The figure shows three views and two pictorial views of one solid part (mm, origin at its lowest corner). Answer the questions. Coordinates: 2 decimals unless noted, no trailing zeros. Loops run counter-clockwise (first coordinate to the right, second up) from the corner with the lowest first, then second, coordinate; pieces in that order, holes last. Notation, with made-up numbers: (76, -20) - (87, -20) arc R21 cw to (87, 16) - close; hole circle Ø9 at (32.5, 58). An arc over 180 degrees is marked (long way). Return JSON: item names as keys, results as strings. Group by question number.
1. Find the intervals of material crossed by line 1 along Z through (x, y) = (76.2, 5); line 2 along X through (y, z) = (4.75, 25.4); line 3 along X through (y, z) = (5, 40.5), in increasing order.
2. Section D-D (y = 2.25) is taken. Write down the section's boundary in (x, z) (1 decimal).
3. Section A-A (x = 63.5) is taken. Write down the section's boundary in (y, z), and give its area (3 significant figures).
4. Section C-C (x = 76.2) is taken. Write down the section's boundary in (y, z), and give its area (3 significant figures).
5. Section B-B (z = 25.4) is taken. Write down the section's boundary in (x, y), and give its area (3 significant figures).
6. This flat-tipped pin is pushed along its axis until it touches: P1, Ø9, axis at x = 50.8, z = 41.275, coming from the -Y side. Where does it stop, or does it pass through?
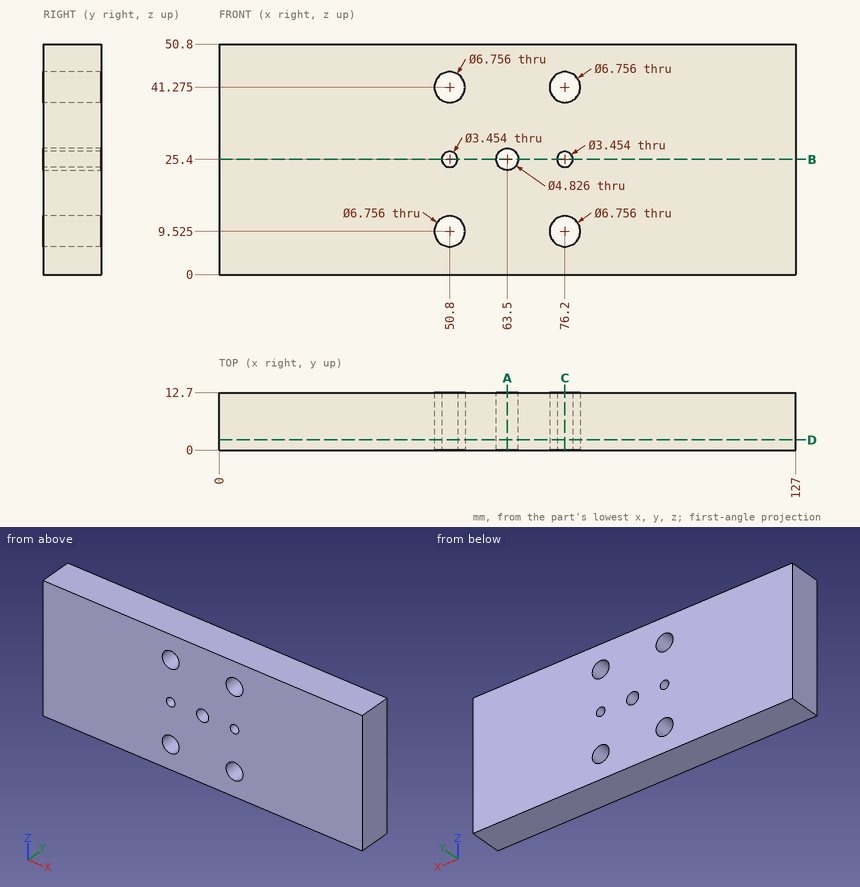
The answers:
{
 "1": {"line 1": "z = 0 to 6.15, 12.9 to 23.67, 27.13 to 37.9, 44.65 to 50.8", "line 2": "x = 0 to 49.07, 52.53 to 61.09, 65.91 to 74.47, 77.93 to 127", "line 3": "x = 0 to 47.51, 54.09 to 72.91, 79.49 to 127"},
 "2": {"outline": "(0, 0) - (127, 0) - (127, 50.8) - (0, 50.8) - close; hole circle Ø6.8 at (50.8, 9.5); hole circle Ø6.8 at (50.8, 41.3); hole circle Ø3.5 at (50.8, 25.4); hole circle Ø4.8 at (63.5, 25.4); hole circle Ø6.8 at (76.2, 9.5); hole circle Ø6.8 at (76.2, 41.3); hole circle Ø3.5 at (76.2, 25.4)"},
 "3": {"outline": "(0, 0) - (12.7, 0) - (12.7, 22.99) - (0, 22.99) - close; (0, 27.81) - (12.7, 27.81) - (12.7, 50.8) - (0, 50.8) - close", "area": "584 mm2"},
 "4": {"outline": "(0, 0) - (12.7, 0) - (12.7, 6.15) - (0, 6.15) - close; (0, 12.9) - (12.7, 12.9) - (12.7, 23.67) - (0, 23.67) - close; (0, 27.13) - (12.7, 27.13) - (12.7, 37.9) - (0, 37.9) - close; (0, 44.65) - (12.7, 44.65) - (12.7, 50.8) - (0, 50.8) - close", "area": "430 mm2"},
 "5": {"outline": "(0, 0) - (49.07, 0) - (49.07, 12.7) - (0, 12.7) - close; (52.53, 0) - (61.09, 0) - (61.09, 12.7) - (52.53, 12.7) - close; (65.91, 0) - (74.47, 0) - (74.47, 12.7) - (65.91, 12.7) - close; (77.93, 0) - (127, 0) - (127, 12.7) - (77.93, 12.7) - close", "area": "1,460 mm2"},
 "6": {"P1": "stops at y = 0"}
}
